Autodesk Inventor part; units mm, degrees
ref_plane "Work Plane1" through (29, 0, 0) normal (0, -1, 0) x (1, 0, 0)
ref_plane "YZ Plane" through (0, 0, 0) normal (1, 0, 0) x (0, 1, 0)
ref_plane "XZ Plane" through (0, 0, 0) normal (0, 1, 0) x (-1, 0, 0)
sketch "Sketch1" plane through (0, 0, 0) normal (0, 0, 1) x (1, 0, 0)
  line L0 (-1.3333, 0) -> (60, 0)
  line L1 (60, 0) -> (60, 3)
  line L2 (60, 3) -> (42, 3)
  line L3 (42, 3) -> (41.3865, 3)
  line L4 (41.3865, 3) -> (0, 3)
  line L5 (0, 3) -> (0, 5)
  line L6 (0, 5) -> (-6, 5)
  line L7 (-6, 5) -> (-6, 2.8868)
  line L8 (-6, 2.8868) -> (-3, 2.8868)
  line L9 (-3, 2.8868) -> (-1.3333, 0)
  line L10 (-19.2, 0) -> (73.2, 0)
  line L11 (0, -1) -> (0, 6)
  line L12 (42, 3) -> (0, 3) construction
  dimension "d1" = 18
  dimension "d2" = 0.6136
  dimension "d3" = 6
  dimension "d4" = 3
  dimension "d5" = 60
  dimension "d6" = 6
  dimension "d7" = 6
  dimension "d8" = 5.7735
  dimension "d9" = 10
  dimension "d26" = 60
revolve "Body" add sketch "Sketch1" angle 360 about axis through (-1.3333, 0, 0) along (1, 0, 0)
sketch "Sketch2" plane through (-6, 0, 0) normal (-1, 0, 0) x (0, 0, 1)
  circle A0 centre (0, 0) radius 2.8868
  line L0 (0, -7) -> (0, 7)
  line L1 (-7, 0) -> (7, 0)
  line L2 (2.8868, 0) -> (1.4434, -2.5)
  line L3 (1.4434, -2.5) -> (-1.4434, -2.5)
  line L4 (-1.4434, -2.5) -> (-2.8868, 0)
  line L5 (-2.8868, 0) -> (-1.4434, 2.5)
  line L6 (-1.4434, 2.5) -> (1.4434, 2.5)
  line L7 (1.4434, 2.5) -> (2.8868, 0)
extrude "Slot" add sketch "Sketch2" against normal up to next contours L7 A0 | A0 L2 | L6 L0 A0 | A0 L0 L3 | L0 L6 A0 | A0 L3 L0 | L4 A0 | A0 L5
fillet "Fillet1" radius 0.6 1 edges at (-6, -5, 0)
thread "Thread"
chamfer "Chamfer1" distance 0.6135 distance2 0.6135 1 edges at (60, -3, 0) measured on face at (60, 1.5134, 0.7943)
ref_plane "Work Plane1" through (29, 0, 0) normal (0, -1, 0) x (1, 0, 0)
fillet "Fillet2" radius 0.1 1 edges at (0, -3, 0)
equation "\"d1\" = GEL"
equation "\"d3\" = KOH"
equation "\"d4\" = INTI"
equation "\"d6\" = GD"
equation "\"d7\" = BDM"
equation "\"d8\" = 1.1547 * SW"
equation "\"d9\" = KOD"
equation "\"d26\" = NLG"
equation "\"d30\" = R"
equation "\"d17\" = RR"
equation "\"d13\" = GEL"
equation "\"d15\" = -0.5 * SPD + 0.5 * GD"
equation "\"d16\" = GUL"
equation "\"GD\" = NND"
equation "\"NLG\" = 60"
equation "\"GEL\" = 18"
equation "\"KOD\" = 10"
equation "\"KOH\" = NND"
equation "\"INTI\" = 3"
equation "\"GAL\" = 0.61345 * PTC"
equation "\"GUL\" = 0.61345 * PTC"
equation "\"BDM\" = NND"
equation "\"SW\" = 5"
equation "\"RR\" = 0.1 * NND"
equation "\"SPD\" = NND - 1.2269 * PTC"
equation "\"R\" = 0.1"
equation "\"PHH\" = 0.2"
equation "\"GD1\" = THREADDIA - 1.2269 * PTC"
equation "\"THREADDIA\" = 6"
equation "\"FAWI\" = 45deg"
equation "\"PTC\" = 1"
equation "\"KOH1\" = 5.4"
equation "\"NND\" = 6"
equation "\"TOA\" = 30deg"
equation "\"E0\" = 1.155 * SW"
properties part number "AS 1420 - 1973 - M6 x 60" material "Steel, Mild"
For this review, take the finished solid that the model builds, in its own axes (mm). A direction names the side the tool comes from. Round coordinates to 2 decimals unless told otherwise and drop trailing zeros. Write each loop counter-clockwise with the first axis right and the second up, starting at its lowest first coordinate (ties: lowest second). Pieces come first, ordered by that corner, then holes. Notation, with made-up numbers: (83.5, 68) - (119.5, 68) arc R29 cw to (119.5, 97) - close; hole circle Ø1 at (-10.75, 21). An arc over 180 degrees is marked (long way). Write each question's results on one line, items separated by ' | '.
Item 1: For faces 1 (the face through (29, -3, 0)), 2 (the face through (60, 0, 0)), 3 (the face through (-4.411, -1.233, 2.175)), list the 3-axis set-ups (+Z, -Z, +X, -X, +Y, -Y) from which the entire face can be reached by the end or side of a thin tool; tool diameter is ignored.
Calculated:
face 1: +X | face 2: +Z, -Z, +X, +Y, -Y | face 3: -X
Item 2: To check wall thickness, follow line 1 along Y through (x, z) = (30, 0.25); line 2 along X through (y, z) = (-1.5, -3.25). State the ranges of each line that lie inside material, in increasing order. Write a range as from..to.
Calculated:
line 1: y = -2.99..2.99 | line 2: x = -6..0
Item 3: For pin 1 (3 mm diameter, centred on x = 20.5, y = -3, fed in from +Z); pin 2 (6 mm diameter, centred on x = 33, z = 0.5, fed in from +Y); pin 3 (1.4 mm diameter, centred on x = -4, z = 0.5, fed in from -Y); pin 4 (1.5 mm diameter, centred on x = 31, y = 3, fed in from -Z), all flat-tipped, find the tip position at first contact; note any pin that passes through.
Calculated:
pin 1: stops at z = 2.6 | pin 2: stops at y = 3 | pin 3: stops at y = -5 | pin 4: stops at z = -1.98
Item 4: Take a section at A-A on x = 15. State the section outline as (y, z) points.
Calculated:
outline: circle Ø6 at (0, 0)
Item 5: Draft analysis for pull direction Z (two halves, no side actions). For faces 4 (the face through (-2.74, -1.08, 4.88)), 5 (the face through (-4.411, -1.268, -2.155)), 6 (the face through (0, 3.3, 0.1)), state which applies: pulls with the +Z half, pulls with the -Z half, needs draft (parallel to the pull), parting line crosses it, or undercut.
Calculated:
face 4: parting line crosses it | face 5: undercut | face 6: needs draft
